Check sheet for the modelled part. Datum: model origin and axes. Units: mm. Face numbers are marked on the shaded views. A direction names the side the tool comes from. Round coordinates to 2 decimals unless told otherwise and drop trailing zeros. Write each loop counter-clockwise with the first axis right and the second up, starting at its lowest first coordinate (ties: lowest second). Pieces come first, ordered by that corner, then holes. Notation, with made-up numbers: (29, -21.5) -> (65, -21.5) arc R16 cw to (65, -6.5) -> close; hole circle Ø9 at (-37.75, -24.75). An arc over 180 degrees is marked (long way). One line per item, written item: value.
from build123d import *

# Parameters (mm, degrees)
SKETCH1_W           = 17.5
SKETCH1_H           = 7.5
SKETCH1_R           = 1
SKETCH1_W_2         = 8.5
SKETCH1_H_2         = 3.5
BOSS_EXTRUDE1_DEPTH = 8
FILLET1_R           = 3
SKETCH3_R           = 1.5
SKETCH3_W           = 2.5
SKETCH3_H           = 1.5
CUT_EXTRUDE1_DEPTH  = 1.5


with BuildPart() as part:
    # Sketch1 → Boss-Extrude1 (new body)
    with BuildSketch(Plane(origin=(0, 0, 0), x_dir=(1, 0, 0), z_dir=(0, 1, 0))):
        Rectangle(SKETCH1_W, SKETCH1_H)
        with Locations((-6.75, 0)):
            Circle(SKETCH1_R, mode=Mode.SUBTRACT)
        with Locations((6.75, 0)):
            Circle(SKETCH1_R, mode=Mode.SUBTRACT)
        Rectangle(SKETCH1_W_2, SKETCH1_H_2, mode=Mode.SUBTRACT)
    extrude(amount=BOSS_EXTRUDE1_DEPTH)

    # Fillet1
    fillet1_edges = [part.edges().sort_by_distance(p)[0] for p in [
        (8.75, 4, 3.75),
        (-8.75, 4, 3.75),
        (-8.75, 4, -3.75),
        (8.75, 4, -3.75),
    ]]
    fillet(fillet1_edges, radius=FILLET1_R)

    # Sketch3 → Cut-Extrude1 (cut)
    with BuildSketch(Plane(origin=(0, 0, 1.75), x_dir=(-1, 0, 0), z_dir=(0, 0, -1))):
        with Locations((0, 6.5)):
            Circle(SKETCH3_R)
        with Locations((0, 7.25)):
            Rectangle(SKETCH3_W, SKETCH3_H)
    cut_extrude1 = extrude(amount=-CUT_EXTRUDE1_DEPTH, mode=Mode.SUBTRACT)

    # Mirror1: Cut-Extrude1 across plane
    add(cut_extrude1.mirror(Plane.XY), mode=Mode.SUBTRACT)


solid = part.part
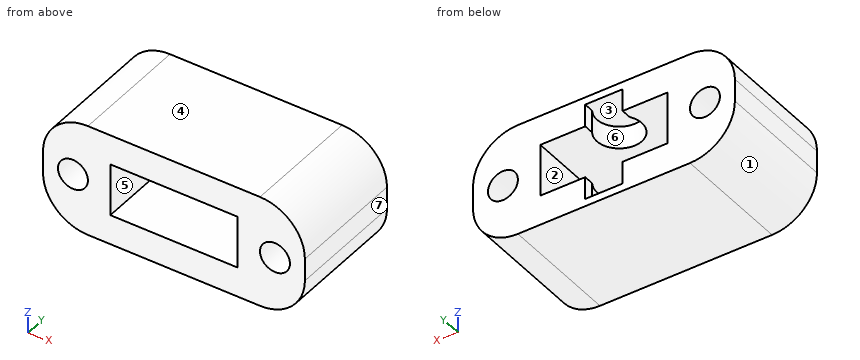
Item 1: Sectioned sample at D-D on z = -1.5. Enter the section's corners in (x, y).
Answer:
outline: (-8.65, 0) -> (-4.25, 0) -> (-4.25, 8) -> (-8.65, 8) -> close; (4.25, 0) -> (8.65, 0) -> (8.65, 8) -> (4.25, 8) -> close
Item 2: Sectioned sample at B-B on y = 3.75. Enter the section's corners in (x, z).
Answer:
outline: (-8.75, -0.75) arc R3 ccw to (-5.75, -3.75) -> (5.75, -3.75) arc R3 ccw to (8.75, -0.75) -> (8.75, 0.75) arc R3 ccw to (5.75, 3.75) -> (-5.75, 3.75) arc R3 ccw to (-8.75, 0.75) -> close; hole circle Ø2 at (-6.75, 0); hole (-4.25, -1.75) -> (4.25, -1.75) -> (4.25, 1.75) -> (-4.25, 1.75) -> close; hole circle Ø2 at (6.75, 0)
Item 3: Tool access check on the marked faces 5, 6 and 7. Record the directions out of +Z, -Z, +X, -X, +Y, -Y that give a thin tool (end or side, any length) a straight path to the whole face; none if there is none.
Answer:
face 5: +Y, -Y
face 6: none
face 7: +Z, -Z, +X, +Y, -Y
Item 4: Thickness scan on line 1 (X direction, y = 4.5, z = 0); line 2 (Z direction, x = -2, y = 7.25); line 3 (Z direction, x = 1, y = 6.5). Record the ranges inside material, lowest first.
Answer:
line 1: x = -8.75 to -7.75, -5.75 to -4.25, 4.25 to 5.75, 7.75 to 8.75
line 2: z = -3.75 to -1.75, 1.75 to 3.75
line 3: z = -3.75 to -3.25, 3.25 to 3.75
Item 5: Sectioned sample at A-A on x = -7.25. Enter the section's corners in (y, z).
Answer:
outline: (0, -3.35) -> (8, -3.35) -> (8, -0.87) -> (0, -0.87) -> close; (0, 0.87) -> (8, 0.87) -> (8, 3.35) -> (0, 3.35) -> close
Item 6: Depth check by flat-ended pin: P1, Ø0.7, axis at y = 7.5, z = -2, coming from the +X side; P2, Ø0.7, axis at y = 8, z = 3, coming from the -X side; P3, Ø0.7, axis at y = 7.5, z = 2.5, coming from the +X side. Enter the tip coordinate at first touch or a pass-through.
Answer:
P1: stops at x = 8.61
P2: stops at x = -8.07
P3: stops at x = 8.4
Item 7: Mould release check, pull along Z, two halves, no side actions. Record for the marked faces 1, 2, 3 and 4: pulls with the +Z half, pulls with the -Z half, needs draft (parallel to the pull), parting line crosses it, or undercut.
Answer:
face 1: pulls with the -Z half
face 2: undercut
face 3: undercut
face 4: pulls with the +Z half
Item 8: Sectioned sample at C-C on z = -0.5. Enter the section's corners in (x, y).
Answer:
outline: (-8.75, 0) -> (-7.62, 0) -> (-7.62, 8) -> (-8.75, 8) -> close; (-5.88, 0) -> (-4.25, 0) -> (-4.25, 8) -> (-5.88, 8) -> close; (4.25, 0) -> (5.88, 0) -> (5.88, 8) -> (4.25, 8) -> close; (7.62, 0) -> (8.75, 0) -> (8.75, 8) -> (7.62, 8) -> close
